```python
from build123d import *

# Parameters (mm, degrees)
ESQUISSE1_R             = 8
ESQUISSE1_R_2           = 4
BOSS_EXTRU_1_DEPTH      = 30
ESQUISSE2_R             = 11
ENL_V_MAT_EXTRU_1_DEPTH = 33.062439084
BOSS_EXTRU_2_START      = 20
ESQUISSE3_R             = 8
ESQUISSE3_R_2           = 4
BOSS_EXTRU_2_DEPTH      = 20


with BuildPart() as part:
    # Esquisse1 → Boss.-Extru.1 (new body)
    with BuildSketch(Plane(origin=(0, 0, 0), x_dir=(1, 0, 0), z_dir=(0, 1, 0))):
        with Locations(Location((0, 0, 0), (0, 0, 270))):
            Circle(ESQUISSE1_R)
        with Locations(Location((0, 0, 0), (0, 0, 270))):
            Circle(ESQUISSE1_R_2, mode=Mode.SUBTRACT)
    extrude(amount=BOSS_EXTRU_1_DEPTH)

    # Esquisse2 → Enlèv. mat.-Extru.1 (cut, through all)
    with BuildSketch(Plane.XY):
        with Locations((0, 15)):
            Circle(ESQUISSE2_R)
    extrude(amount=-ENL_V_MAT_EXTRU_1_DEPTH, mode=Mode.SUBTRACT)

    # Esquisse3 → Boss.-Extru.2 (add)
    with BuildSketch(Plane.XZ.offset(BOSS_EXTRU_2_START)):
        with Locations(Location((0, 0, 0), (0, 0, 270))):
            Circle(ESQUISSE3_R)
        with Locations(Location((0, 0, 0), (0, 0, 270))):
            Circle(ESQUISSE3_R_2, mode=Mode.SUBTRACT)
    extrude(amount=-BOSS_EXTRU_2_DEPTH)


solid = part.part
```
For this review, take the finished solid that the model builds, in its own axes (mm). A direction names the side the tool comes from. Give positions to 0.01 mm unless a question says otherwise; leave off trailing zeros. Write each loop counter-clockwise with the first axis right and the second up, starting at its lowest first coordinate (ties: lowest second). Pieces come first, ordered by that corner, then holes. Notation, with made-up numbers: M 33,-37 L 79,-37 A16 cw 79,-17 Z; hole C 7.25,-29 d3. An arc over 180 degrees is marked long. One line per item, written item: value.
1) Take a section at A-A, the plane x = 0. Write out the cut boundary in (y, z).
Results are:
outline: M -20,-8 L 4,-8 L 4,-4 L -20,-4 Z; M -20,4 L 30,4 L 30,8 L -20,8 Z; M 26,-8 L 30,-8 L 30,-4 L 26,-4 Z
2) Take a section at C-C, the plane y = -15.5. Write out the cut boundary in (x, z), then the cut area to 3 significant figures.
Results are:
outline: C 0,0 d16; hole C 0,0 d8
area: 151 mm²
3) Take a section at B-B, the plane z = -3.5. Write out the cut boundary in (x, y).
Results are:
outline: M -7.19,-20 L -1.94,-20 L -1.94,4.17 A11 cw -7.19,6.68 Z; M -7.19,23.32 A11 cw -1.94,25.83 L -1.94,30 L -7.19,30 Z; M 1.94,-20 L 7.19,-20 L 7.19,6.68 A11 cw 1.94,4.17 Z; M 1.94,25.83 A11 cw 7.19,23.32 L 7.19,30 L 1.94,30 Z
4) For P1, Ø5, axis at y = -2, z = 6, coming from the +X side; P2, Ø8, axis at x = 0, z = -3, coming from the -Y side; P3, Ø5, axis at x = 3, y = 16.5, coming from the +Z side; P4, Ø3, axis at x = 6.5, y = 17, coming from the -Z side, all flat-tipped, find the tip position at first contact; note any pin that passes through.
Results are:
P1: stops at x = 7.19
P2: stops at y = -20
P3: stops at z = 7.98
P4: stops at z = 0
5) For faces 1 (the flat face through (-2, 30, -4)), 2 (the flat face through (-6, 15, 0)), list the 3-axis set-ups (+Z, -Z, +X, -X, +Y, -Y) from which the entire face can be reached by the end or side of a thin tool; tool diameter is ignored.
Results are:
face 1: +Z, -Z, +X, -X, +Y
face 2: -Z
6) Take a section at D-D, the plane x = 5.5. Write out the cut boundary in (y, z), then the cut area to 3 significant figures.
Results are:
outline: M -20,-5.81 L 5.47,-5.81 L 5.47,0 L 24.53,0 L 24.53,-5.81 L 30,-5.81 L 30,5.81 L -20,5.81 Z
area: 470 mm²
7) The part is to be moulded in two halves that separate along X. For faces 3 (the flat face through (-2, -20, 4)), 4 (the cylindrical face through (0, 4, -5)), say which applies: +X half, -X half, draft (parallel to the pull), parting line (faces both ways), or undercut.
Results are:
face 3: draft
face 4: undercut
8) For line 1 (X direction, y = -10.5, z = 0); line 2 (Z direction, x = -2.75, y = 26), list the stretches that pass through material, from the lowest coordinate up. Write a range as from..to.
Results are:
line 1: x = -8..-4, 4..8
line 2: z = -7.51..-2.9, 2.9..7.51
